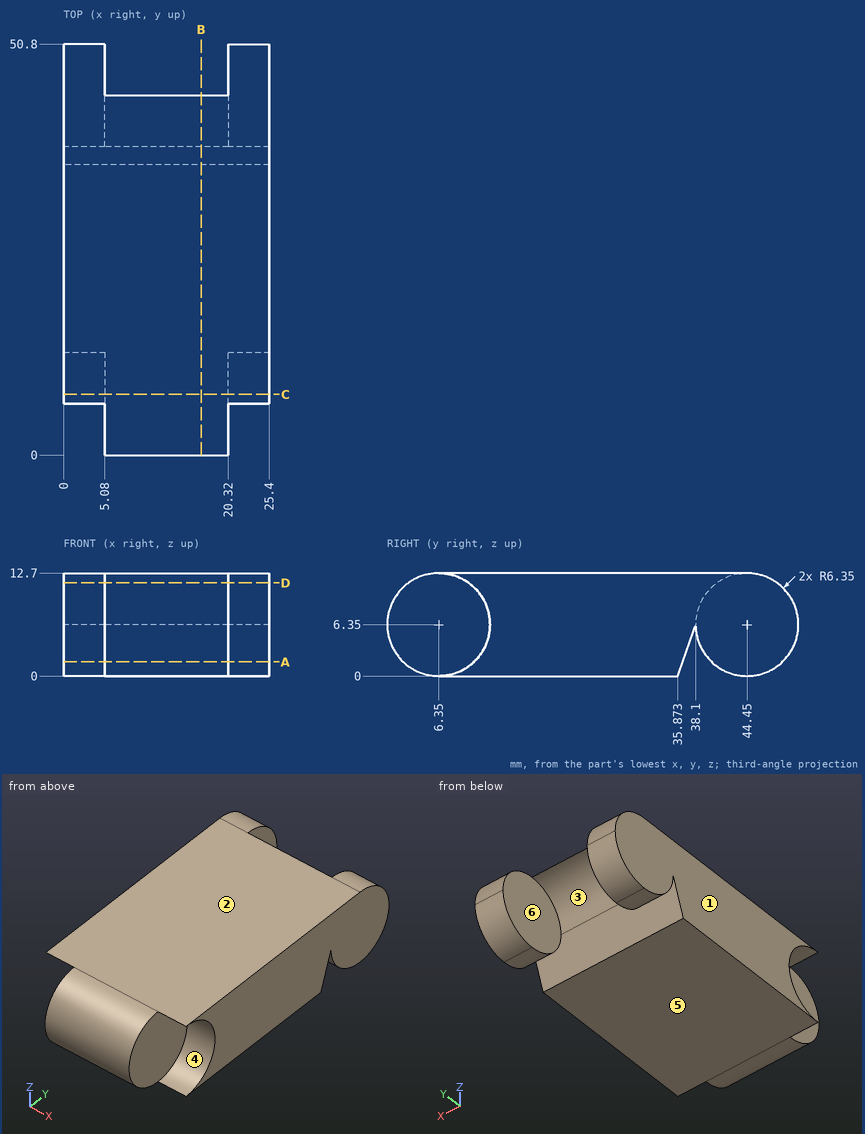
Study the drawing (mm; zero at the part's minimum x, y, z) and answer. A direction names the side the tool comes from. Give positions to 0.01 mm unless a question says otherwise; leave off trailing zeros. Write each loop counter-clockwise with the first axis right and the second up, starting at its lowest first coordinate (ties: lowest second). Pieces come first, ordered by that corner, then holes. Notation, with made-up numbers: M 9.5,84.25 L 29.5,84.25 A18 ccw 29.5,119.25 Z; hole C 2,-14 d3. An arc over 180 degrees is marked long. Put each result on its own line as item: value. Start each with the question number.
1. The part is cut by section A-A, the plane z = 1.75. Give the vertices of the cut face in (x, y).
2. Which of the six approach directions +Z, -Z, +X, -X, +Y, -Y give full straight-line access (tool end or side, diameter ignored) to the marked faces 4, 5 and 6?
3. The part is cut by section D-D, the plane z = 11.5. Give the vertices of the cut face in (x, y) (3 decimals).
4. Each of these flat-tipped pins is pushed along its axis until it touches: pin 1 Ø6.5 at (y, z) = (5.5, 4.5) entering from -X; pin 2 Ø4 at (y, z) = (42.5, 7.5) entering from -X. Where does it stop, or does it pass through?
5. Consider line 1 along X through (y, z) = (41, 7.75); line 2 along Y through (x, z) = (2.5, 5.5); line 3 along X through (y, z) = (12, 6). Determine where each line is inside the solid, lowest interval first.
6. The part is cut by section B-B, the plane x = 17. Give the vertices of the cut face in (y, z).
7. For a pull along X with two mould halves and no side action, classify the marked faces 1, 2 and 3 as released by +X, released by -X, zero draft, split by the parting line, or undercut.
8. The part is cut by section C-C, the plane y = 7.5. Give the vertices of the cut face in (x, z) (3 decimals), and give its area (3 significant figures).
Final values:
1. outline: M 0,10.73 L 5.08,10.73 L 5.08,1.97 L 20.32,1.97 L 20.32,10.73 L 25.4,10.73 L 25.4,36.49 L 0,36.49 Z; M 0,40.07 L 5.08,40.07 L 5.08,48.83 L 0,48.83 Z; M 20.32,40.07 L 25.4,40.07 L 25.4,48.83 L 20.32,48.83 Z
2. face 4: +X, -Y
2. face 5: -Z, +X, -X, +Y, -Y
2. face 6: -Z, +Y
3. outline: M 0,10.065 L 5.08,10.065 L 5.08,2.635 L 20.32,2.635 L 20.32,10.065 L 25.4,10.065 L 25.4,48.165 L 20.32,48.165 L 20.32,40.735 L 5.08,40.735 L 5.08,48.165 L 0,48.165 Z
4. pin 1: stops at x = 5.08
4. pin 2: stops at x = 0
5. line 1: x = 0 to 5.08, 20.32 to 25.4
5. line 2: y = 12.64 to 37.8, 38.16 to 50.74
5. line 3: x = 5.08 to 20.32
6. outline: M 6.35,0 L 35.87,0 L 38.1,6.35 A6.35 cw 44.45,12.7 L 6.35,12.7 A6.35 ccw Z
7. face 1: released by -X
7. face 2: zero draft
7. face 3: undercut
8. outline: M 0,0 L 25.4,0 L 25.4,0.105 L 20.32,0.105 L 20.32,12.595 L 25.4,12.595 L 25.4,12.7 L 0,12.7 L 0,12.595 L 5.08,12.595 L 5.08,0.105 L 0,0.105 Z
8. area: 196 mm²
